Autodesk Inventor part; units mm, degrees
ref_plane "YZ Plane" through (0, 0, 0) normal (1, 0, 0) x (0, 1, 0)
ref_plane "XZ Plane" through (0, 0, 0) normal (0, 1, 0) x (-1, 0, 0)
ref_plane "XY Plane" through (0, 0, 0) normal (0, 0, 1) x (1, 0, 0)
sketch "main" plane through (0, 0, 0) normal (0, 0, 1) x (1, 0, 0)
  circle A0 centre (31.4944, -42.9627) radius 2.1844
  arc A1 (31.4944, -49.3127) -> (37.0053, -39.8078) centre (31.4944, -42.9627) ccw
  arc A2 (-34.551, -37.1452) -> (-32.0056, -49.3127) centre (-32.0056, -42.9627) ccw
  arc A3 (-34.551, -37.1452) -> (17.2626, -11.6066) centre (-289.0911, 544.606) ccw
  line L0 (37.0053, -39.8078) -> (21.5498, -12.8103)
  line L1 (-32.0056, -49.3127) -> (31.4944, -49.3127)
  arc A4 (21.5498, -12.8103) -> (17.2626, -11.6066) centre (18.7944, -14.3877) ccw
  circle A5 centre (-32.0056, -42.9627) radius 2.0955
  point P0 (5.1717, -33.3366)
  point P1 (19.9944, -10.0932)
  dimension "d0" = 1270
  dimension "d1" = 12.7
  dimension "d2" = 12.7
  dimension "d3" = 3.175
  dimension "d4" = 4.191
  dimension "d7" = 34.925
  dimension "d8" = 12.7
sketch "Sketch1" plane through (0, 0, 0) normal (0, 1, 0) x (-1, 0, 0)
  circle A0 centre (-0.1035, -63.4999) radius 2.1844
  arc A1 (-6.4535, -63.4896) -> (3.0424, -69.0159) centre (-0.1035, -63.4999) ccw
  arc A2 (5.8217, 2.5359) -> (-6.35, 0.0103) centre (0, 0) ccw
  arc A3 (5.8217, 2.5359) -> (31.2757, -49.3193) centre (587.9868, 256.1277) ccw
  line L0 (3.0424, -69.0159) -> (30.0651, -53.6045)
  line L1 (-6.35, 0.0103) -> (-6.4535, -63.4896)
  arc A4 (30.0651, -53.6045) -> (31.2757, -49.3193) centre (28.4922, -50.8465) ccw
  circle A5 centre (0, 0) radius 2.0955
  point P0 (0, 0)
extrude "Extrusion1" add sketch "Sketch1" along normal blind 1.5875
properties part number "Magazine Gusset" material "Acetal Resin, White"
Design review of the part built by this model. Coordinates are the model's own, in mm. Give positions to 0.01 mm unless a question says otherwise; leave off trailing zeros. Loops run counter-clockwise (first coordinate to the right, second up) from the corner with the lowest first, then second, coordinate; pieces in that order, holes last. Notation, with made-up numbers: (59.25, 80) -> (76.25, 80) arc R18 cw to (76.25, 110) -> close; hole circle Ø7 at (63, -28). An arc over 180 degrees is marked (long way). Write each question's results on one line, items separated by ' | '.
Q1. Wall thickness on L1, parallel to Z at x = 0, y = 0.6; L2, parallel to X at y = 0.1, z = -64; L3, parallel to Z at x = -29, y = 1.45: over which ranges is each line inside the solid? List them lowest first.
Reply:
L1: z = -69.85 to -65.68, -61.32 to -2.1, 2.1 to 6.35 | L2: x = -11.84 to -2.02, 2.23 to 6.43 | L3: z = -54.21 to -45.13
Q2. Take a section at C-C, the plane z = -16. Write out the cut boundary in (x, y).
Reply:
outline: (-14.25, 0) -> (6.38, 0) -> (6.38, 1.59) -> (-14.25, 1.59) -> close
Q3. Take a section at B-B, the plane x = 0. Write out the cut boundary in (y, z), plus the area to 3 significant figures.
Reply:
outline: (0, -69.85) -> (1.59, -69.85) -> (1.59, -65.68) -> (0, -65.68) -> close; (0, -61.32) -> (1.59, -61.32) -> (1.59, -2.1) -> (0, -2.1) -> close; (0, 2.1) -> (1.59, 2.1) -> (1.59, 6.35) -> (0, 6.35) -> close | area: 107 mm²
Q4. The part is to be moulded in two halves that separate along X. For faces 1 (the face through (0.388, 0.783, -65.666)), 2 (the face through (-18.137, 0.783, -24.044)), 3 (the face through (-8, 0, -31)), say which applies: +X half, -X half, draft (parallel to the pull), parting line (faces both ways), or undercut.
Reply:
face 1: undercut | face 2: -X half | face 3: draft
Q5. Take a section at D-D, the plane x = -21. Write out the cut boundary in (y, z), plus the area to 3 significant figures.
Reply:
outline: (0, -58.77) -> (1.59, -58.77) -> (1.59, -29.79) -> (0, -29.79) -> close | area: 46.0 mm²
Q6. Take a section at A-A, the plane y = 0.4. Write out the cut boundary in (x, z), plus the area to 3 significant figures.
Reply:
outline: (-31.28, -49.32) arc R3.17 ccw to (-30.07, -53.6) -> (-3.04, -69.02) arc R6.35 ccw to (6.45, -63.49) -> (6.35, 0.01) arc R6.35 ccw to (-5.82, 2.54) arc R635.04 cw to start; hole circle Ø4.19 at (0, 0); hole circle Ø4.37 at (0.1, -63.5) | area: 1,790 mm²
